```python
from build123d import *

# Parameters (mm, degrees)
SKETCH1_W           = 70
SKETCH1_H           = 30
BOSS_EXTRUDE1_DEPTH = 20
CUT_EXTRUDE1_REACH  = 52.249
SKETCH2_R           = 5
SKETCH3_R           = 2
BOSS_EXTRUDE2_DEPTH = 5
DOME1_FACE_RADIUS   = 2
DOME1_HEIGHT        = 8
DOME2_FACE_RADIUS   = 2
DOME2_HEIGHT        = 8


with BuildPart() as part:
    # Sketch1 → Boss-Extrude1 (new body)
    with BuildSketch(Plane(origin=(0, 0, 0), x_dir=(1, 0, 0), z_dir=(0, 1, 0))):
        Rectangle(SKETCH1_W, SKETCH1_H)
    extrude(amount=BOSS_EXTRUDE1_DEPTH)

    # Sketch2 → Cut-Extrude1 (cut, up to next)
    with BuildSketch(Plane(origin=(0, 0, -15), x_dir=(-1, 0, 0), z_dir=(0, 0, -1)), mode=Mode.PRIVATE) as cut_extrude1_sk1:
        with Locations((-25, 10)):
            Circle(SKETCH2_R)
    cut_extrude1_tool1 = extrude(cut_extrude1_sk1.sketch, amount=-CUT_EXTRUDE1_REACH, mode=Mode.PRIVATE) & part.part
    # Sketch2 → Cut-Extrude1 (cut, up to next)
    with BuildSketch(Plane(origin=(0, 0, -15), x_dir=(-1, 0, 0), z_dir=(0, 0, -1)), mode=Mode.PRIVATE) as cut_extrude1_sk2:
        with Locations((25, 10)):
            Circle(SKETCH2_R)
    cut_extrude1_tool2 = extrude(cut_extrude1_sk2.sketch, amount=-CUT_EXTRUDE1_REACH, mode=Mode.PRIVATE) & part.part
    add(cut_extrude1_tool1.solids().sort_by_distance((25, 10, -15))[0], mode=Mode.SUBTRACT)
    add(cut_extrude1_tool2.solids().sort_by_distance((-25, 10, -15))[0], mode=Mode.SUBTRACT)

    # Sketch3 → Boss-Extrude2 (add)
    with BuildSketch(Plane(origin=(0, 20, 0), x_dir=(1, 0, 0), z_dir=(0, 1, 0))):
        with Locations(Location((-25, 0, 0), (0, 0, 270))):
            Circle(SKETCH3_R)
        with Locations(Location((25, 0, 0), (0, 0, 270))):
            Circle(SKETCH3_R)
    extrude(amount=BOSS_EXTRUDE2_DEPTH)

    # Dome1: a dome of height H over a round flat face of radius A is a cap of a sphere of radius (A * A + H * H) / (2 * H)
    dome1_r = (DOME1_FACE_RADIUS * DOME1_FACE_RADIUS + DOME1_HEIGHT * DOME1_HEIGHT) / (2 * DOME1_HEIGHT)
    dome1_base = Plane((-25, 25, 0), z_dir=(0, 1, 0))
    with Locations(dome1_base.offset(DOME1_HEIGHT - dome1_r)):
        dome1_ball = Sphere(dome1_r, mode=Mode.PRIVATE)
    add(split(dome1_ball, bisect_by=dome1_base, keep=Keep.TOP, mode=Mode.PRIVATE))

    # Dome2: a dome of height H over a round flat face of radius A is a cap of a sphere of radius (A * A + H * H) / (2 * H)
    dome2_r = (DOME2_FACE_RADIUS * DOME2_FACE_RADIUS + DOME2_HEIGHT * DOME2_HEIGHT) / (2 * DOME2_HEIGHT)
    dome2_base = Plane((25, 25, 0), z_dir=(0, 1, 0))
    with Locations(dome2_base.offset(DOME2_HEIGHT - dome2_r)):
        dome2_ball = Sphere(dome2_r, mode=Mode.PRIVATE)
    add(split(dome2_ball, bisect_by=dome2_base, keep=Keep.TOP, mode=Mode.PRIVATE))


solid = part.part
```
CAD build for the part. Positions are in the model's coordinates, mm. A direction names the side the tool comes from. Give positions to 0.01 mm unless a question says otherwise; leave off trailing zeros. Loops run counter-clockwise (first coordinate to the right, second up) from the corner with the lowest first, then second, coordinate; pieces in that order, holes last. Notation, with made-up numbers: (49, -25.5) -> (70, -25.5) arc R12 ccw to (70, -21.5) -> close; hole circle Ø1 at (84, 12.25). An arc over 180 degrees is marked (long way). Use a Markdown table: item, result.
1. Mould opens along Y. For faces 1 (the flat face through (35, 10, 0)), 2 (the flat face through (0, 0, 0)), 3 (the cylindrical face through (23, 22, 0)) say: pulls with the +Y half, pulls with the -Y half, needs draft (parallel to the pull), parting line crosses it, or undercut.
Check result:
| item | result |
|---|---|
| face 1 | needs draft |
| face 2 | pulls with the -Y half |
| face 3 | undercut |
2. Which spindle directions (+Z, -Z, +X, -X, +Y, -Y) get a long thin tool onto all of the face, cutting with end or side? Do faces 4 (the cylindrical face through (-20, 10, 0)), 5 (the cylindrical face through (-26.2, 22.5, -1.6)). Say none if no direction does.
Check result:
| item | result |
|---|---|
| face 4 | +Z, -Z |
| face 5 | none |
3. Flat gauge pin, fed straight in: pin 1 (9 mm diameter, centred on x = -25, y = 10, fed in from -Z). Where does the tip first touch, or does it go through?
Check result:
| item | result |
|---|---|
| pin 1 | passes through |
4. Slice it at B-B (y = 14). List the corners of the cut face in (x, z), plus the area to 3 significant figures.
Check result:
| item | result |
|---|---|
| outline | (-35, -15) -> (-28, -15) -> (-28, 15) -> (-35, 15) -> close; (-22, -15) -> (22, -15) -> (22, 15) -> (-22, 15) -> close; (28, -15) -> (35, -15) -> (35, 15) -> (28, 15) -> close |
| area | 1,740 mm^2 |
5. Slice it at A-A (x = 25). List the corners of the cut face in (y, z), plus the area to 3 significant figures.
Check result:
| item | result |
|---|---|
| outline | (0, -15) -> (5, -15) -> (5, 15) -> (0, 15) -> close; (15, -15) -> (20, -15) -> (20, -2) -> (25, -2) arc R4.25 ccw (long way) to (25, 2) -> (20, 2) -> (20, 15) -> (15, 15) -> close |
| area | 375 mm^2 |
6. Slice it at D-D (y = 10). List the corners of the cut face in (x, z), plus the area to 3 significant figures.
Check result:
| item | result |
|---|---|
| outline | (-35, -15) -> (-30, -15) -> (-30, 15) -> (-35, 15) -> close; (-20, -15) -> (20, -15) -> (20, 15) -> (-20, 15) -> close; (30, -15) -> (35, -15) -> (35, 15) -> (30, 15) -> close |
| area | 1,500 mm^2 |
7. Slice it at C-C (z = 0). List the corners of the cut face in (x, y), plus the area to 3 significant figures.
Check result:
| item | result |
|---|---|
| outline | (-35, 0) -> (35, 0) -> (35, 20) -> (27, 20) -> (27, 25) arc R4.25 ccw (long way) to (23, 25) -> (23, 20) -> (-23, 20) -> (-23, 25) arc R4.25 ccw (long way) to (-27, 25) -> (-27, 20) -> (-35, 20) -> close; hole circle Ø10 at (-25, 10); hole circle Ø10 at (25, 10) |
| area | 1,390 mm^2 |
8. Wall check: L1, parallel to Y at x = -25, z = -0.25; L2, parallel to Y at x = -25, z = -3.75; L3, parallel to Y at x = 25, z = -4.5. Give the ranges that are in metal, low to high. Write a range as [from, to].
Check result:
| item | result |
|---|---|
| L1 | y = [0, 5], [15, 32.99] |
| L2 | y = [0, 5], [15, 20], [26.75, 30.75] |
| L3 | y = [0, 5], [15, 20] |
